Verification items for the finished model (mm, model axes). Give positions to 0.01 mm unless a question says otherwise; leave off trailing zeros. Write each loop counter-clockwise with the first axis right and the second up, starting at its lowest first coordinate (ties: lowest second). Pieces come first, ordered by that corner, then holes. Notation, with made-up numbers: (-16, -0.5) -> (22, -0.5) arc R11 ccw to (22, 17.5) -> close; hole circle Ø4 at (24, 60). An arc over 180 degrees is marked (long way). Answer as CSV lines item,"result". Start each with the question number.
1) Material ranges on L1, parallel to Z at x = 35.25, y = -0.3; L2, parallel to Z at x = 34, y = -0.65; L3, parallel to X at y = -0.2, z = -4, recorded low to high.
2) Sectioned sample at C-C on y = -0.6. Record the cut outline in (x, z), and give its area (3 significant figures).
3) Sectioned sample at B-B on z = -5.5. Record the cut outline in (x, y).
4) Mould release check, pull along Z, two halves, no side actions. Record for faces 1 (the flat face through (-0.6, 0, 9.3)), 2 (the cylindrical face through (13.764, -0.493, 0.057)): released by +Z, released by -Z, zero draft, split by the parting line, or undercut.
5) Sectioned sample at D-D on z = 16.75. Record the cut outline in (x, y).
6) Gauge pin test, flat end, axial feed: pin 1 Ø3.5 at (x, z) = (-15.06, 0) entering from -Y. Record the tip position at first contact, or that the pin passes through.
7) Sectioned sample at A-A on x = -25.55. Record the cut outline in (y, z), and give its area (3 significant figures).
```python
from build123d import *

# Parameters (mm, degrees)
SKETCH_W                  = 81.5
SKETCH_H                  = 40.5
SKETCH_R                  = 1.89865
SKETCH_R_2                = 1.3
SKETCH_W_2                = 23
SKETCH_H_2                = 18
EXTRUDE001_DEPTH          = 1
FILLET_R                  = 1
FILLET001_R               = 1
FILLET001_PLACEMENT_ANGLE = 90


with BuildPart() as part:
    # Sketch → Extrude001 (new body)
    with BuildSketch(Plane.XY):
        Rectangle(SKETCH_W, SKETCH_H)
        with Locations((-36.35, 15.65)):
            Circle(SKETCH_R, mode=Mode.SUBTRACT)
        with Locations((-25.55, 16.75)):
            Circle(SKETCH_R, mode=Mode.SUBTRACT)
        with Locations((35.25, -16.15)):
            Circle(SKETCH_R, mode=Mode.SUBTRACT)
        with Locations((35.25, 15.85)):
            Circle(SKETCH_R, mode=Mode.SUBTRACT)
        with Locations((-15.0625, 0)):
            Circle(SKETCH_R_2, mode=Mode.SUBTRACT)
        with Locations((15.0625, 0)):
            Circle(SKETCH_R_2, mode=Mode.SUBTRACT)
        Rectangle(SKETCH_W_2, SKETCH_H_2, mode=Mode.SUBTRACT)
    extrude(amount=EXTRUDE001_DEPTH)

    # Fillet
    fillet_edges = [part.edges().sort_by_distance(p)[0] for p in [
        (-40.75, 20.25, 0.5),
        (40.75, 20.25, 0.5),
        (40.75, -20.25, 0.5),
        (-40.75, -20.25, 0.5),
    ]]
    fillet(fillet_edges, radius=FILLET_R)

    # Fillet001
    fillet001_edges = [part.edges().sort_by_distance(p)[0] for p in [
        (-11.5, 9, 0.5),
        (11.5, 9, 0.5),
        (11.5, -9, 0.5),
        (-11.5, -9, 0.5),
    ]]
    fillet(fillet001_edges, radius=FILLET001_R)


with BuildPart() as part_1:
    # Fillet001 placement: moved
    add(part.part.rotate(Axis((0, 0, 0), (1, 0, 0)), FILLET001_PLACEMENT_ANGLE))


solid = part_1.part
```
Ans:
1,L1,"z = -20.25 to -18.05, -14.25 to 13.95, 17.75 to 20.25"
1,L2,"z = -20.25 to -17.58, -14.72 to 14.42, 17.28 to 20.25"
1,L3,"x = -40.75 to -11.5, 11.5 to 40.75"
2,outline,"(-40.75, -19.25) arc R1 ccw to (-39.75, -20.25) -> (39.75, -20.25) arc R1 ccw to (40.75, -19.25) -> (40.75, 19.25) arc R1 ccw to (39.75, 20.25) -> (-39.75, 20.25) arc R1 ccw to (-40.75, 19.25) -> close; hole circle Ø3.8 at (-36.35, 15.65); hole circle Ø3.8 at (-25.55, 16.75); hole circle Ø2.6 at (-15.06, 0); hole (-11.5, -8) arc R1 ccw to (-10.5, -9) -> (10.5, -9) arc R1 ccw to (11.5, -8) -> (11.5, 8) arc R1 ccw to (10.5, 9) -> (-10.5, 9) arc R1 ccw to (-11.5, 8) -> close; hole circle Ø2.6 at (15.06, 0); hole circle Ø3.8 at (35.25, -16.15); hole circle Ø3.8 at (35.25, 15.85)"
2,area,"2,830 mm²"
3,outline,"(-40.75, -1) -> (-11.5, -1) -> (-11.5, 0) -> (-40.75, 0) -> close; (11.5, -1) -> (40.75, -1) -> (40.75, 0) -> (11.5, 0) -> close"
4,face 1,"zero draft"
4,face 2,"undercut"
5,outline,"(-40.75, -1) -> (-37.9, -1) -> (-37.9, 0) -> (-40.75, 0) -> close; (-34.8, -1) -> (-27.45, -1) -> (-27.45, 0) -> (-34.8, 0) -> close; (-23.65, -1) -> (33.58, -1) -> (33.58, 0) -> (-23.65, 0) -> close; (36.92, -1) -> (40.75, -1) -> (40.75, 0) -> (36.92, 0) -> close"
6,pin 1,"stops at y = -1"
7,outline,"(-1, -20.25) -> (0, -20.25) -> (0, 14.85) -> (-1, 14.85) -> close; (-1, 18.65) -> (0, 18.65) -> (0, 20.25) -> (-1, 20.25) -> close"
7,area,"36.7 mm²"
